The listing builds one solid part. Answer for the finished solid, in the listing's coordinates (mm). Face numbers are marked on the shaded views. A direction names the side the tool comes from. Coordinates: 2 decimals unless noted, no trailing zeros. Loops run counter-clockwise (first coordinate to the right, second up) from the corner with the lowest first, then second, coordinate; pieces in that order, holes last. Notation, with made-up numbers: (62, -20) - (75, -20) arc R20 ccw to (75, 1) - close; hole circle Ø11 at (77, 5). An arc over 180 degrees is marked (long way). Return JSON: item names as keys, results as strings. Group by question number.
1. Find the intervals of material crossed by line 1 along X through (y, z) = (19.75, 3); line 2 along X through (y, z) = (12, 34); line 3 along Z through (x, y) = (-30, 14.25), in increasing order.
2. The mould has two halves that part along Z. Classify the marked faces 4, 5 and 6: pulls with the +Z half, pulls with the -Z half, needs draft (parallel to the pull), parting line crosses it, or undercut.
3. Each of these flat-tipped pins is pushed along its axis until it touches: P1, Ø8, axis at y = 12, z = 13, coming from the -X side; P2, Ø8.5, axis at x = 35.56, y = 22.62, coming from the +Z side; P3, Ø12.5, axis at y = 16, z = 14, coming from the +X side. Where does it stop, or does it pass through?
4. Section D-D (x = -19.5) is taken. Write down the section's boundary in (y, z), and give its area (3 significant figures).
5. Which of the six approach directions +Z, -Z, +X, -X, +Y, -Y give full straight-line access (tool end or side, diameter ignored) to the marked faces 1, 2 and 3?
6. Section C-C (z = 8) is taken. Write down the section's boundary in (x, y), and give its area (3 significant figures).
7. Section A-A (x = -30.48) is taken. Write down the section's boundary in (y, z), and give its area (3 significant figures).
8. Section B-B (y = 9.25) is taken. Write down the section's boundary in (x, z).
```python
from build123d import *

# Parameters (mm, degrees)
SKETCH1_R             = 3.175
BOSS_EXTRUDE9_DEPTH   = 3.048
BOSS_EXTRUDE9_2_DEPTH = 3.048
SKETCH1_17_W          = 5.08
SKETCH1_17_H          = 24.892
BOSS_EXTRUDE10_DEPTH  = 38.1
FILLET3_R             = 2.54
FILLET4_R             = 2.54
FILLET6_R             = 12.446
SKETCH2_R             = 4.953
CUT_EXTRUDE1_DEPTH    = 38.1


with BuildPart() as part:
    # Sketch1 → Boss-Extrude9 (new body)
    with BuildSketch(Plane.XY):
        with BuildLine():
            Line((0, 2.809544612), (0, 27.701544612))
            Line((0, 27.701544612), (-33.02, 27.701544612))
            ThreePointArc((-33.02, 27.701544612), (-34.816051224, 26.957595836), (-35.56, 25.161544612))
            Line((-35.56, 25.161544612), (-35.56, 5.349544612))
            ThreePointArc((-35.56, 5.349544612), (-34.816051224, 3.553493388), (-33.02, 2.809544612))
            Line((-33.02, 2.809544612), (0, 2.809544612))
        make_face()
        with Locations(Location((-30.48, 7.889544612, 0), (0, 0, 180))):
            Circle(SKETCH1_R, mode=Mode.SUBTRACT)
        with Locations(Location((-30.48, 22.621544612, 0), (0, 0, 180))):
            Circle(SKETCH1_R, mode=Mode.SUBTRACT)
    extrude(amount=BOSS_EXTRUDE9_DEPTH)



with BuildPart() as body_2:
    # Sketch1 → Boss-Extrude9 2 (new body)
    with BuildSketch(Plane.XY):
        with BuildLine():
            Line((38.1, 27.701544612), (5.08, 27.701544612))
            Line((5.08, 27.701544612), (5.08, 2.809544612))
            Line((5.08, 2.809544612), (38.1, 2.809544612))
            ThreePointArc((38.1, 2.809544612), (39.896051224, 3.553493388), (40.64, 5.349544612))
            Line((40.64, 5.349544612), (40.64, 25.161544612))
            ThreePointArc((40.64, 25.161544612), (39.896051224, 26.957595836), (38.1, 27.701544612))
        make_face()
        with Locations(Location((35.56, 7.889544612, 0), (0, 0, 180))):
            Circle(SKETCH1_R, mode=Mode.SUBTRACT)
        with Locations(Location((35.56, 22.621544612, 0), (0, 0, 180))):
            Circle(SKETCH1_R, mode=Mode.SUBTRACT)
    extrude(amount=BOSS_EXTRUDE9_2_DEPTH)


with BuildPart() as part_1:
    add(part.part)

    add(body_2.part)  # Boss-Extrude10 merges body 2
    # Sketch1<17> → Boss-Extrude10 (add)
    with BuildSketch(Plane.XY):
        with Locations((2.54, 15.255544612)):
            Rectangle(SKETCH1_17_W, SKETCH1_17_H)
    extrude(amount=BOSS_EXTRUDE10_DEPTH)

    # Fillet3
    fillet3_edges = [part_1.edges().sort_by_distance(p)[0] for p in [
        (5.08, 15.255544612, 3.048),
    ]]
    fillet(fillet3_edges, radius=FILLET3_R)

    # Fillet4
    fillet4_edges = [part_1.edges().sort_by_distance(p)[0] for p in [
        (0, 15.255544612, 3.048),
    ]]
    fillet(fillet4_edges, radius=FILLET4_R)

    # Fillet6
    fillet6_edges = [part_1.edges().sort_by_distance(p)[0] for p in [
        (2.54, 2.809544612, 38.1),
        (2.54, 27.701544612, 38.1),
    ]]
    fillet(fillet6_edges, radius=FILLET6_R - 0.0001)  # a hair under: the kernel refuses the full size

    # Sketch2 → Cut-Extrude1 (cut)
    with BuildSketch(Plane.ZY):
        with Locations(Location((26.501688995, 15.255544612, 0), (0, 0, 270))):
            Circle(SKETCH2_R)
    extrude(amount=-CUT_EXTRUDE1_DEPTH, mode=Mode.SUBTRACT)


solid = part_1.part
```
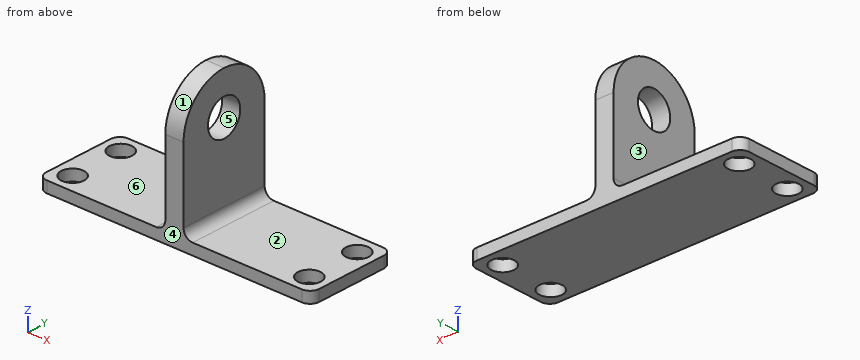
The answers:
{
 "1": {"line 1": "x = -35.56 to -31.83, -29.13 to 34.21, 36.91 to 40.64", "line 2": "x = 0 to 5.08", "line 3": "z = 0 to 3.05"},
 "2": {"face 4": "needs draft", "face 5": "undercut", "face 6": "pulls with the +Z half"},
 "3": {"P1": "stops at x = 0", "P2": "stops at z = 3.05", "P3": "stops at x = 5.08"},
 "4": {"outline": "(2.81, 0) - (27.7, 0) - (27.7, 3.05) - (2.81, 3.05) - close", "area": "75.9 mm2"},
 "5": {"face 1": "+Z, +X, -X, -Y", "face 2": "+Z, +X, +Y, -Y", "face 3": "+Z, -X, +Y, -Y"},
 "6": {"outline": "(0, 2.81) - (5.08, 2.81) - (5.08, 27.7) - (0, 27.7) - close", "area": "126 mm2"},
 "7": {"outline": "(2.81, 0) - (4.71, 0) - (4.71, 3.05) - (2.81, 3.05) - close; (11.06, 0) - (19.45, 0) - (19.45, 3.05) - (11.06, 3.05) - close; (25.8, 0) - (27.7, 0) - (27.7, 3.05) - (25.8, 3.05) - close", "area": "37.2 mm2"},
 "8": {"outline": "(-35.56, 0) - (-33.35, 0) - (-33.35, 3.05) - (-35.56, 3.05) - close; (-27.61, 0) - (32.69, 0) - (32.69, 3.05) - (7.62, 3.05) arc R2.54 cw to (5.08, 5.59) - (5.08, 36.56) - (0, 36.56) - (0, 5.59) arc R2.54 cw to (-2.54, 3.05) - (-27.61, 3.05) - close; (38.43, 0) - (40.64, 0) - (40.64, 3.05) - (38.43, 3.05) - close"}
}
